Answer from the drawing. Dimensions are ordinates in mm from the lowest x, y and z of the part. A direction names the side the tool comes from. Give positions to 0.01 mm unless a question says otherwise; leave off trailing zeros. Write each loop counter-clockwise with the first axis right and the second up, starting at its lowest first coordinate (ties: lowest second). Pieces come first, ordered by that corner, then holes. Notation, with made-up numbers: (-2.5, -13) -> (54.5, -13) arc R32 ccw to (54.5, 13) -> close; hole circle Ø2 at (28.5, -12). An arc over 180 degrees is marked (long way). Use a Markdown table: item, result. Add a question column.
Q1. For a pull along Z with two mould halves and no side action, classify the marked faces 1, 2, 3 and 4 as pulls with the +Z half, pulls with the -Z half, needs draft (parallel to the pull), parting line crosses it, or undercut.
Q2. Section C-C, the plane x = 5 is taken. Give the vertices of the cut face in (y, z), plus the area to 3 significant figures.
Q3. Section B-B, the plane y = 41 is taken. Give the vertices of the cut face in (x, z).
Q4. Each of these flat-tipped pins is pushed along its axis until it touches: pin 1 Ø5 at (y, z) = (37, 42) entering from +X; pin 2 Ø9.5 at (x, y) = (22.5, 22) entering from -Z; pin 3 Ø8 at (x, y) = (29.5, 36.5) entering from +Z; pin 4 Ø3 at (x, z) = (5, 5) entering from -Y. Where does it stop, or does it pass through?
Q5. Section A-A, the plane z = 42 is taken. Give the vertices of the cut face in (x, y).
Q6. Section D-D, the plane y = 12.5 is taken. Give the vertices of the cut face in (x, z), plus the area to 3 significant figures.
Q7. For the marked faces 5, 6, 7 and 8, determine the directions among +Z, -Z, +X, -X, +Y, -Y from which every point of the face is accessible in a straight line to the end or side of a thin tool.
Q8. Consider line 1 (Z direction, x = 5, y = 43); line 2 (Z direction, x = 44.5, y = 37); line 3 (Y direction, x = 15.25, z = 42). Determine where each line is inside the solid, lowest interval first.
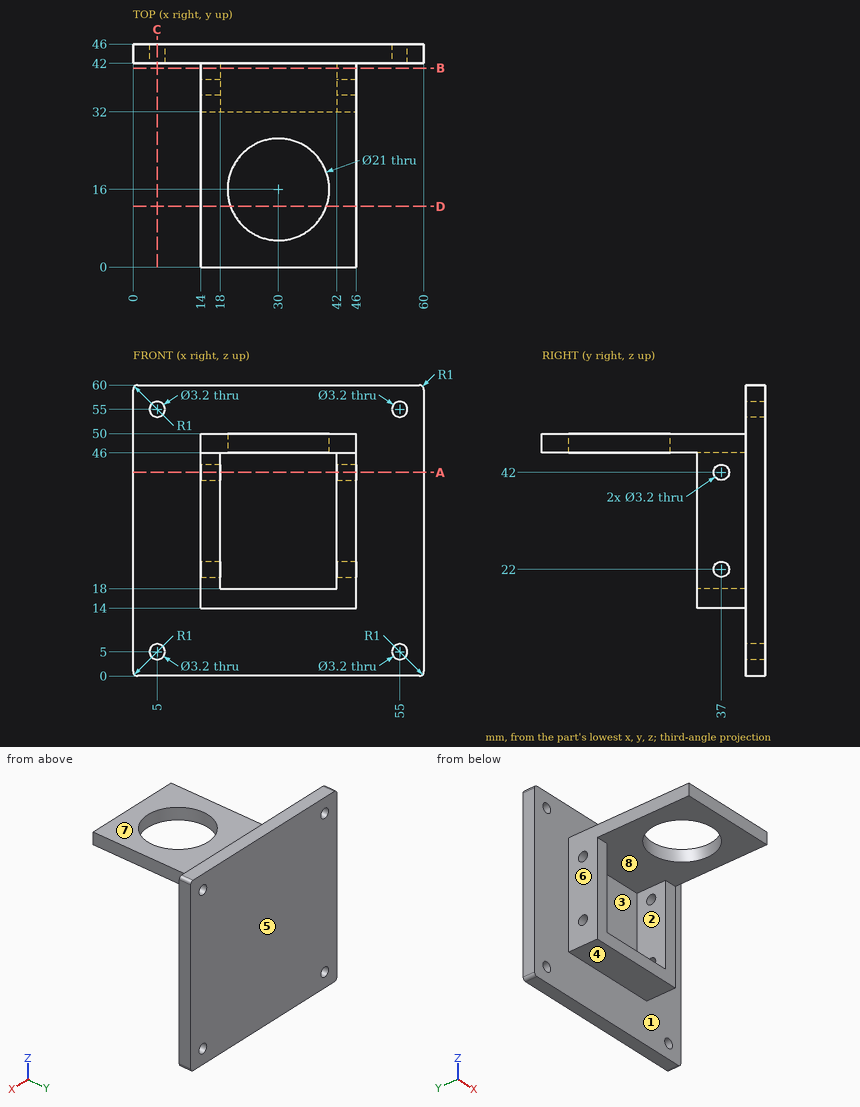
Result set:
| question | item | result |
|---|---|---|
| 1 | face 1 | needs draft |
| 1 | face 2 | undercut |
| 1 | face 3 | undercut |
| 1 | face 4 | pulls with the -Z half |
| 2 | outline | (42, 0) -> (46, 0) -> (46, 3.4) -> (42, 3.4) -> close; (42, 6.6) -> (46, 6.6) -> (46, 53.4) -> (42, 53.4) -> close; (42, 56.6) -> (46, 56.6) -> (46, 60) -> (42, 60) -> close |
| 2 | area | 214 mm2 |
| 3 | outline | (14, 14) -> (46, 14) -> (46, 50) -> (14, 50) -> close; hole (18, 18) -> (42, 18) -> (42, 46) -> (18, 46) -> close |
| 4 | pin 1 | stops at x = 46 |
| 4 | pin 2 | stops at z = 46 |
| 4 | pin 3 | stops at z = 50 |
| 4 | pin 4 | passes through |
| 5 | outline | (0, 42) -> (14, 42) -> (14, 38.6) -> (18, 38.6) -> (18, 42) -> (42, 42) -> (42, 38.6) -> (46, 38.6) -> (46, 42) -> (60, 42) -> (60, 46) -> (0, 46) -> close; (14, 32) -> (18, 32) -> (18, 35.4) -> (14, 35.4) -> close; (42, 32) -> (46, 32) -> (46, 35.4) -> (42, 35.4) -> close |
| 6 | outline | (14, 46) -> (20.1, 46) -> (20.1, 50) -> (14, 50) -> close; (39.9, 46) -> (46, 46) -> (46, 50) -> (39.9, 50) -> close |
| 6 | area | 48.8 mm2 |
| 7 | face 5 | +Z, -Z, +X, -X, +Y |
| 7 | face 6 | +Z, -Z, -X, -Y |
| 7 | face 7 | +Z, +X, -X, -Y |
| 7 | face 8 | -Y |
| 8 | line 1 | z = 0 to 3.4, 6.6 to 53.4, 56.6 to 60 |
| 8 | line 2 | z = 14 to 20.4, 23.6 to 40.4, 43.6 to 50 |
| 8 | line 3 | y = 32 to 35.4, 38.6 to 46 |
